Work out the finished part from the listing and answer in its coordinate system (mm). Face numbers are marked on the shaded views. A direction names the side the tool comes from. Coordinates: 2 decimals unless noted, no trailing zeros. Write each loop counter-clockwise with the first axis right and the second up, starting at its lowest first coordinate (ties: lowest second). Pieces come first, ordered by that corner, then holes. Notation, with made-up numbers: M 58.25,-24.5 L 114.25,-24.5 A9 ccw 114.25,-10.5 Z; hole C 72,67.5 d2. An arc over 180 degrees is marked long. Answer as CSV lines item,"result". Start each with the question number.
(1) Find the intervals of material crossed by L1, parallel to X at y = -9.5, z = 3.2; L2, parallel to Y at x = 77, z = 1.1; L3, parallel to Y at x = 5.5, z = 3.55, in increasing order. Write a range as [from, to].
(2) A cutting plane is placed at D-D on z = 3.1. Count the separate pieces of the cut face and the enclosed holes in it, then the cut area to 3 significant figures.
(3) The mould has two halves that part along X. Classify the marked faces 1, 2 and 3: released by +X, released by -X, zero draft, split by the parting line, or undercut.
(4) A cutting plane is placed at B-B on x = 103.5. Give the vertices of the cut face in (y, z).
(5) A cutting plane is placed at C-C on x = 37.5. Give the vertices of the cut face in (y, z).
(6) For the marked faces 4, 5 and 6, determine the directions among +Z, -Z, +X, -X, +Y, -Y from which every point of the face is accessible in a straight line to the end or side of a thin tool.
(7) Flat-ended cylindrical pins translate along their axes: P1, Ø8, axis at x = 110.5, y = 6, coming from the -Z side; P2, Ø0.5, axis at y = 22.5, z = 2.5, coming from the +X side; P3, Ø3, axis at y = -8, z = 2, coming from the -X side; P4, Ø4, axis at x = 111, y = -2.5, coming from the -Z side. Find the tip coordinate at first contact, or state that the pin passes through.
(8) A cutting plane is placed at A-A on x = 5.5. Give the vertices of the cut face in (y, z), then the cut area to 3 significant figures.
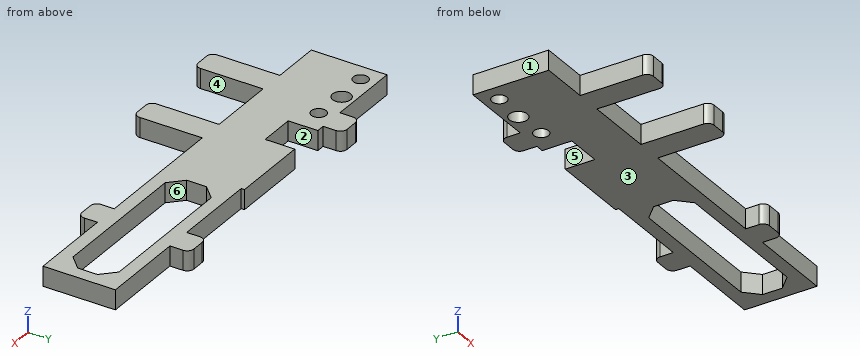
Autodesk Inventor part; units mm, degrees
ref_plane "YZ Plane" through (0, 0, 0) normal (1, 0, 0) x (0, 1, 0)
ref_plane "XZ Plane" through (0, 0, 0) normal (0, 1, 0) x (-1, 0, 0)
ref_plane "XY Plane" through (0, 0, 0) normal (0, 0, 1) x (1, 0, 0)
sketch "Sketch1" plane through (0, 0, 0) normal (0, 0, 1) x (1, 0, 0)
  line L0 (0, 0) -> (128, 0)
  line L1 (128, 0) -> (128, 22)
  line L2 (0, 23) -> (0, 0)
  line L3 (68, 23) -> (68, 22)
  line L4 (68, 22) -> (128, 22)
  line L5 (33, 23) -> (33, 14)
  line L6 (33, 14) -> (44, 14)
  line L7 (44, 14) -> (44, 23)
  line L8 (68, 23) -> (44, 23)
  line L9 (33, 23) -> (0, 23)
  line L10 (72, 14) -> (72, 8)
  line L11 (72, 8) -> (76, 4)
  line L12 (76, 4) -> (120, 4)
  line L13 (120, 4) -> (124, 8)
  line L14 (124, 8) -> (124, 14)
  line L15 (124, 14) -> (120, 18)
  line L16 (120, 18) -> (76, 18)
  line L17 (76, 18) -> (72, 14)
  line L18 (68, 22) -> (68, 0) construction
  circle A0 centre (5.5, 18.5) radius 2.25
  circle A1 centre (25.5, 18.5) radius 2.25
  circle A2 centre (15.5, 19.099) radius 2.75
  circle A3 centre (38.5, 19.099) radius 7.5 construction
  circle A4 centre (38.5, 19.099) radius 4 construction
  point P0 (33, 18.5)
  dimension "d0" = 128
  dimension "d1" = 23
  dimension "d2" = 22
  dimension "d3" = 60
  dimension "d4" = 11
  dimension "d5" = 9
  dimension "d6" = 33
  dimension "d7" = 45
  dimension "d8" = 4
  dimension "d9" = 4
  dimension "d10" = 4
  dimension "d11" = 4
  dimension "d12" = 4
  dimension "d13" = 4.5
  dimension "d14" = 4.5
  dimension "d15" = 5.5
  dimension "d16" = 20
  dimension "d17" = 5.5
  dimension "d18" = 8
  dimension "d19" = 15
  dimension "d20" = 10
extrude "Extrusion1" add sketch "Sketch1" along normal blind 6
sketch "Sketch2" plane through (0, 0, 6) normal (0, 0, 1) x (1, 0, 0)
  line L0 (0, 0) -> (128, 0)
  line L1 (128, 0) -> (128, 22)
  line L2 (128, 22) -> (68, 22)
  line L3 (33, 23) -> (0, 23)
  line L4 (0, 23) -> (0, 0)
  line L5 (22.5, 23) -> (30.5, 23)
  line L6 (30.5, 23) -> (30.5, 27)
  line L7 (28.5, 29) -> (24.5, 29)
  line L8 (22.5, 27) -> (22.5, 23)
  line L9 (94, 22) -> (102, 22)
  line L10 (102, 22) -> (102, 26)
  line L11 (100, 28) -> (96, 28)
  line L12 (94, 26) -> (94, 22)
  line L13 (15, 0) -> (23, 0)
  line L14 (23, 0) -> (23, -19)
  line L15 (21, -21) -> (17, -21)
  line L16 (15, -19) -> (15, 0)
  line L17 (44, 0) -> (52, 0)
  line L18 (52, 0) -> (52, -19)
  line L19 (50, -21) -> (46, -21)
  line L20 (44, -19) -> (44, 0)
  line L21 (94, 0) -> (102, 0)
  line L22 (102, 0) -> (102, -4)
  line L23 (100, -6) -> (96, -6)
  line L24 (94, -4) -> (94, 0)
  arc A0 (24.5, 29) -> (22.5, 27) centre (24.5, 27) ccw
  arc A1 (30.5, 27) -> (28.5, 29) centre (28.5, 27) ccw
  arc A2 (96, 28) -> (94, 26) centre (96, 26) ccw
  arc A3 (102, 26) -> (100, 28) centre (100, 26) ccw
  arc A4 (15, -19) -> (17, -21) centre (17, -19) ccw
  arc A5 (21, -21) -> (23, -19) centre (21, -19) ccw
  arc A6 (44, -19) -> (46, -21) centre (46, -19) ccw
  arc A7 (50, -21) -> (52, -19) centre (50, -19) ccw
  arc A8 (94, -4) -> (96, -6) centre (96, -4) ccw
  arc A9 (100, -6) -> (102, -4) centre (100, -4) ccw
  dimension "d23" = 2
  dimension "d24" = 8
  dimension "d25" = 8
  dimension "d26" = 8
  dimension "d27" = 8
  dimension "d28" = 8
  dimension "d29" = 21
  dimension "d30" = 6
  dimension "d31" = 6
  dimension "d32" = 22.5
  dimension "d33" = 26
  dimension "d34" = 15
  dimension "d35" = 21
  dimension "d38" = 6
extrude "Extrusion2" add sketch "Sketch2" against normal blind 6
properties part number "x_iddler_upper_nut_stop"
Here are the results:
1,L1,"x = [15, 23], [44, 52]"
1,L2,"y = [0, 4], [18, 22]"
1,L3,"y = [0, 16.25], [20.75, 23]"
2,separate pieces,"1"
2,enclosed holes,"4"
2,area,"2,500 mm^2"
3,face 1,"released by -X"
3,face 2,"undercut"
3,face 3,"zero draft"
4,outline,"M 0,0 L 4,0 L 4,6 L 0,6 Z; M 18,0 L 22,0 L 22,6 L 18,6 Z"
5,outline,"M 0,0 L 14,0 L 14,6 L 0,6 Z"
6,face 4,"+Z, -Z, -Y"
6,face 5,"+Z, -Z, +Y"
6,face 6,"+Z, -Z"
7,P1,"stops at z = 0"
7,P2,"stops at x = 102"
7,P3,"stops at x = 15"
7,P4,"passes through"
8,outline,"M 0,0 L 16.25,0 L 16.25,6 L 0,6 Z; M 20.75,0 L 23,0 L 23,6 L 20.75,6 Z"
8,area,"111 mm^2"
